Geometry: final body of the model. Coordinates: model frame, mm. Face numbers are marked on the shaded views. Give positions to 0.01 mm unless a question says otherwise; leave off trailing zeros. Write each loop counter-clockwise with the first axis right and the second up, starting at its lowest first coordinate (ties: lowest second). Pieces come first, ordered by that corner, then holes. Notation, with made-up numbers: M -39.75,64 L 6.25,64 A14 cw 6.25,77 Z; hole C 15.5,53 d10. An arc over 180 degrees is marked long. Answer as a JSON object with one key per item and string values.
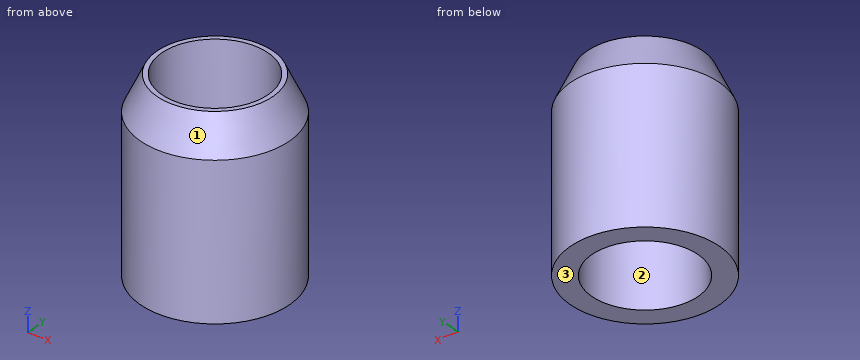
Autodesk Inventor part; units mm, degrees
ref_plane "YZ Plane" through (0, 0, 0) normal (1, 0, 0) x (0, 1, 0)
ref_plane "XZ Plane" through (0, 0, 0) normal (0, 1, 0) x (-1, 0, 0)
ref_plane "XY Plane" through (0, 0, 0) normal (0, 0, 1) x (1, 0, 0)
sketch "Sketch1" plane through (0, 0, 0) normal (0, 0, 1) x (1, 0, 0)
  circle A0 centre (0, 0) radius 15
  circle A1 centre (0, 0) radius 21
  dimension "d0" = 30
  dimension "d1" = 42
extrude "Extrusion1" add sketch "Sketch1" along normal blind 53
sketch "Sketch2" plane through (0, 0, 0) normal (0, 0, -1) x (-1, 0, 0)
  circle A0 centre (0, 0) radius 17.5
  circle A1 centre (0, 0) radius 21
  dimension "d4" = 35
  dimension "d5" = 42
extrude "Extrusion2" add sketch "Sketch2" along normal blind 5
chamfer "Chamfer2" distance 10 angle 25 1 edges at (-21, 0, 53) measured on face at (20.9319, -1.6898, 35.3333)
thicken "Thicken1" operation add thickness 5 both sides no extend neighbours yes toward (0, 0, 1) faces at (-19.4604, -3.0712, -5)
properties part number "Nikon-Objective-Insulation" material "ABS Plastic"
1) Contact query for flat-ended pins moving along their axis: P1, Ø5, axis at x = -6, z = 27.5, coming from the +Y side; P2, Ø12, axis at x = -9.5, y = 4.5, coming from the -Z side; P3, Ø10, axis at x = 3.5, z = 24.5, coming from the +Y side; P4, Ø2, axis at x = 11.5, z = 21.5, coming from the +Y side. Output: stop coordinate, or through.
Geometry check:
{"P1": "stops at y = 20.71", "P2": "stops at z = 0", "P3": "stops at y = 21", "P4": "stops at y = 18.19"}
2) Cut plane A-A on x = 0. Return loops of the section in (y, z).
Geometry check:
{"outline": "M -21,0 L -15,0 L -15,53 L -16.34,53 L -21,43 Z; M 15,0 L 21,0 L 21,43 L 16.34,53 L 15,53 Z"}
3) Cut plane C-C on z = 38. Return loops of the section in (x, y).
Geometry check:
{"outline": "C 0,0 d42; hole C 0,0 d30"}
4) Pull-direction query (X, two-part tool) for the marked faces 1, 2 and 3; classes: pulls with the +X half, pulls with the -X half, needs draft (parallel to the pull), parting line crosses it, or undercut.
Geometry check:
{"face 1": "parting line crosses it", "face 2": "undercut", "face 3": "needs draft"}
5) Line query: line 1 (Y direction, x = 0, z = 42.5); line 2 (Y direction, x = 4.5, z = 49); line 3 (X direction, y = 2.5, z = 21). Output: solid intervals per line, ascending. Write a range as from..to.
Geometry check:
{"line 1": "y = -21..-15, 15..21", "line 2": "y = -17.64..-14.31, 14.31..17.64", "line 3": "x = -20.85..-14.79, 14.79..20.85"}
